Source: three-view drawing plus pictorial views. Frame: mm from the lowest corner of the part. A direction names the side the tool comes from. Give positions to 0.01 mm unless a question says otherwise; leave off trailing zeros. Order: outer loops, then holes, each group sorted by start corner. A loop starts at its lowest first (then second) coordinate and runs counter-clockwise, first axis right, second up. Notation, with made-up numbers: (38, 75) -> (96, 75) arc R7 ccw to (96, 88) -> close; hole circle Ø7 at (-9.75, 44.5). An arc over 180 degrees is marked (long way). Write item = value, one per line.
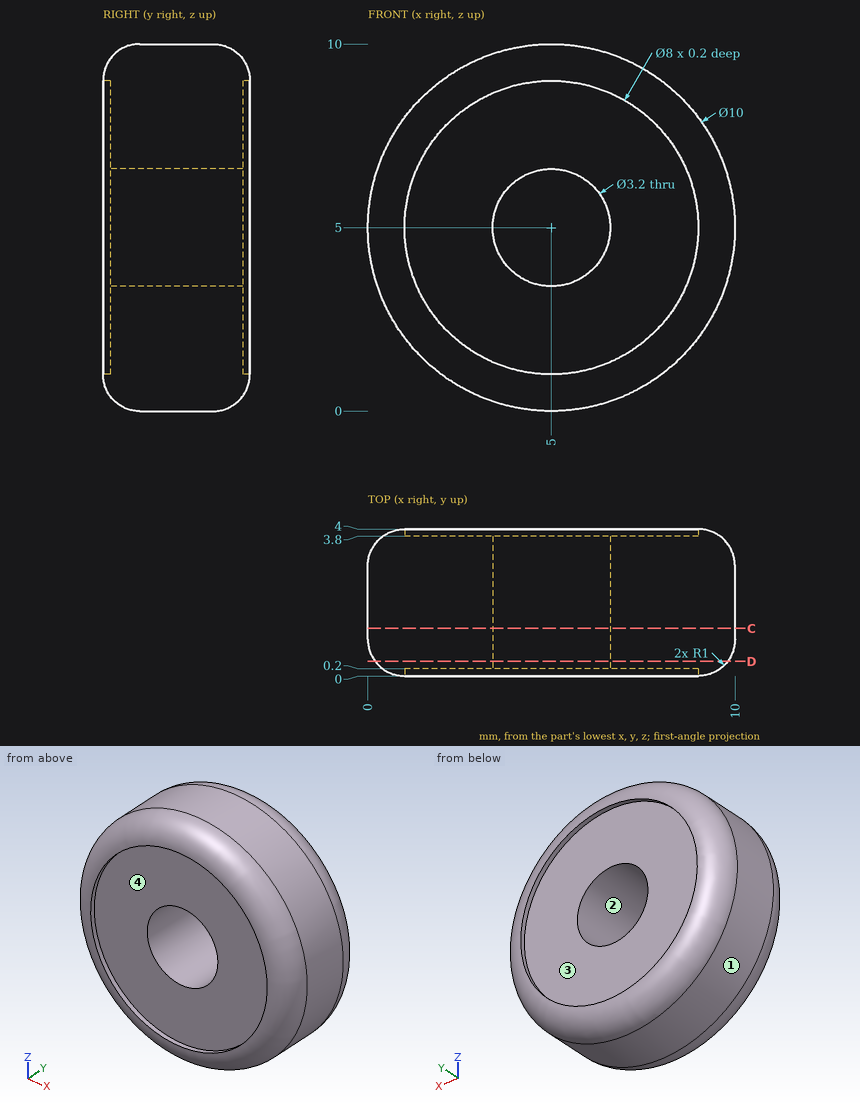
1) Mould query, pull axis X, two halves, no side actions, for the marked faces 1 and 2. Classes: +X half, -X half, draft (parallel to the pull), parting line (faces both ways), or undercut.
Check sheet entries:
face_1 = parting line
face_2 = undercut
2) Reachability of the marked faces 3 and 4 from +Z, -Z, +X, -X, +Y, -Y: full face, straight path, thin tool, end or side. Return the list, or none.
Check sheet entries:
face_3 = +Y
face_4 = -Y
3) Section query D-D (y = 0.4). Output: boundary loops of the cut face in (x, z).
Check sheet entries:
outline = circle Ø9.6 at (5, 5); hole circle Ø3.2 at (5, 5)
4) Section query C-C (y = 1.3). Output: boundary loops of the cut face in (x, z), plus the area to 3 significant figures.
Check sheet entries:
outline = circle Ø10 at (5, 5); hole circle Ø3.2 at (5, 5)
area = 70.5 mm²
5) Line query: line 1 (X direction, y = 1.85, z = 5); line 2 (Y direction, x = 3.25, z = 3.75); line 3 (Z direction, x = 2, y = 2.45). Output: solid intervals per line, ascending. Write a range as from..to.
Check sheet entries:
line_1 = 0..3.4, 6.6..10
line_2 = 0.2..3.8
line_3 = 1..9
6) First-contact query: P1, Ø3, axis at x = 3.5, z = 4, coming from the +Y side; P2, Ø3.5, axis at x = 5, z = 5, coming from the -Y side. Flat tips, straight axial feed; report the tip coordinate or a pass-through.
Check sheet entries:
P1 = 3.8
P2 = 0.2
